Verification items for the finished model (mm, model axes). A direction names the side the tool comes from. Round coordinates to 2 decimals unless told otherwise and drop trailing zeros. Loops run counter-clockwise (first coordinate to the right, second up) from the corner with the lowest first, then second, coordinate; pieces in that order, holes last. Notation, with made-up numbers: (38, -3) - (42, -3) arc R21 cw to (42, 18) - close; hole circle Ø2 at (6.5, 73.5). An arc over 180 degrees is marked (long way). Use a Markdown table: item, result. Add a question column.
Autodesk Inventor part; units mm, degrees
ref_plane "YZ Plane" through (0, 0, 0) normal (1, 0, 0) x (0, 1, 0)
ref_plane "XZ Plane" through (0, 0, 0) normal (0, 1, 0) x (-1, 0, 0)
ref_plane "XY Plane" through (0, 0, 0) normal (0, 0, 1) x (1, 0, 0)
sketch "Sketch1" plane through (0, 0, 0) normal (0, 1, 0) x (-1, 0, 0)
  circle A0 centre (0, 0) radius 42.5
  arc A1 (55.6417, 25) -> (-55.6417, 25) centre (0, 0) ccw
  line L0 (0, 0) -> (0, -61)
  line L1 (0, 0) -> (0, 0)
  line L2 (0, 0) -> (0, -90.4875)
  line L3 (-117.5, 25) -> (-117.5, -25)
  line L4 (117.5, -25) -> (117.5, 25)
  line L5 (117.5, 25) -> (-117.5, -25) construction
  line L6 (-117.5, 25) -> (117.5, -25) construction
  line L7 (117.5, 25) -> (55.6417, 25)
  line L8 (-55.6417, 25) -> (-117.5, 25)
  line L9 (55.6417, -25) -> (117.5, -25)
  line L10 (-117.5, -25) -> (-55.6417, -25)
  arc A2 (-55.6417, -25) -> (55.6417, -25) centre (0, 0) ccw
  dimension "d0" = 85
  dimension "d29" = 61
  dimension "d46" = 235
  dimension "d47" = 50
extrude "Extrusion1" add sketch "Sketch1" along normal blind 5
sketch "Sketch2" plane through (0, 0, 0) normal (0, -1, 0) x (1, 0, 0)
  line L0 (-117.5, -25) -> (-117.5, 25)
  line L1 (-117.5, 0) -> (117.5, 0)
  line L2 (117.5, 25) -> (117.5, -25)
  arc A0 (55.6417, 25) -> (-55.6417, 25) centre (0, 0) ccw
  line L3 (0, 61) -> (0, -61)
  arc A1 (-55.6417, -25) -> (55.6417, -25) centre (0, 0) ccw
  circle A2 centre (-98.5, 11) radius 2
  line L4 (-117.5, 25) -> (-55.6417, 25)
  circle A3 centre (-78.5, 11) radius 2
  circle A4 centre (-98.5, -11) radius 2
  circle A5 centre (-78.5, -11) radius 2
  circle A6 centre (98.5, 11) radius 2
  circle A7 centre (78.5, 11) radius 2
  circle A8 centre (98.5, -11) radius 2
  circle A9 centre (78.5, -11) radius 2
  dimension "d51" = 4
  dimension "d52" = 19
  dimension "d53" = 14
  dimension "d54" = 4
  dimension "d55" = 20
hole "Hole1" at (-98.5, 0, 11) at (-78.5, 0, 11) at (-78.5, 0, -11) at (-98.5, 0, -11) at (78.5, 0, 11) at (98.5, 0, 11) at (98.5, 0, -11) at (78.5, 0, -11) direction (0, 1, 0) diameter 3.242 depth 11.8 tip angle 118
sketch "Sketch3" plane through (0, 0, 0) normal (0, -1, 0) x (1, 0, 0)
  circle A0 centre (0, 0) radius 51
  circle A1 centre (0, 51) radius 2
  circle A2 centre (-44.1673, 25.5) radius 2
  circle A3 centre (-44.1673, -25.5) radius 2
  circle A4 centre (0, -51) radius 2
  circle A5 centre (44.1673, -25.5) radius 2
  circle A6 centre (44.1673, 25.5) radius 2
  dimension "d33" = 102
  dimension "d34" = 4
  dimension "d37" = 360
hole "Hole2" at (0, 0, 51) at (44.1673, 0, 25.5) at (44.1673, 0, -25.5) at (0, 0, -51) at (-44.1673, 0, -25.5) at (-44.1673, 0, 25.5) direction (0, 1, 0) diameter 3.242 depth 11.8 tip angle 118
fillet "Fillet2" radius 5 8 edges at (-117.5, 2.5, -25) (-55.6417, 2.5, -25) (117.5, 2.5, -25) (55.6417, 2.5, -25) (117.5, 2.5, 25) (55.6417, 2.5, 25) (-55.6417, 2.5, 25) (-117.5, 2.5, 25)
properties part number "Head Thing (metal)"
Q1. Section check C-C on x = 4.5. Record the cut outline in (y, z), plus the area to 3 significant figures.
Q2. Section check D-D on x = -94.5. Record the cut outline in (y, z), plus the area to 3 significant figures.
Q3. Set-up check for faces 1 (the face through (-86, 2, 25)), 2 (the face through (85, 2, 25)), 3 (the face through (-85, 2, -25)): record each of +Z, -Z, +X, -X, +Y, -Y from which the full face is reachable in a straight line by a thin tool's end or side.
Q4. Section check B-B on y = 3.25. State how many separate pieces and enclosed holes the cut face has, plus the area to 3 significant figures.
Q5. Go/stop test with flat-tipped pins: pin 1 Ø1.9 at (x, z) = (-78.5, -11) entering from -Y; pin 2 Ø2.5 at (x, y) = (-76, 2.5) entering from -Z; pin 3 Ø1 at (x, y) = (-23, 3.5) entering from -Z; pin 4 Ø2.5 at (x, y) = (93, 1.5) entering from +Z. Record where each tip stops, or that it passes through.
Q6. Thickness scan on line 1 along Z through (x, y) = (98.5, 1.25); line 2 along Z through (x, y) = (0, 1.35); line 3 along X through (y, z) = (1.8, -11). Record the ranges inside material, lowest first.
Q7. Section check A-A on z = 0. Record the cut outline in (x, y), plus the area to 3 significant figures.
Determined:
| question | item | result |
|---|---|---|
| 1 | outline | (0, -60.83) - (5, -60.83) - (5, -42.26) - (0, -42.26) - close; (0, 42.26) - (5, 42.26) - (5, 60.83) - (0, 60.83) - close |
| 1 | area | 186 mm² |
| 2 | outline | (0, -25) - (5, -25) - (5, 25) - (0, 25) - close |
| 2 | area | 250 mm² |
| 3 | face 1 | +Z, -X, +Y, -Y |
| 3 | face 2 | +Z, +X, +Y, -Y |
| 3 | face 3 | -Z, -X, +Y, -Y |
| 4 | separate pieces | 1 |
| 4 | enclosed holes | 15 |
| 4 | area | 11,700 mm² |
| 5 | pin 1 | passes through |
| 5 | pin 2 | stops at z = -25 |
| 5 | pin 3 | stops at z = -56.7 |
| 5 | pin 4 | stops at z = 25 |
| 6 | line 1 | z = -25 to -12.62, -9.38 to 9.38, 12.62 to 25 |
| 6 | line 2 | z = -61 to -52.62, -49.38 to -42.5, 42.5 to 49.38, 52.62 to 61 |
| 6 | line 3 | x = -117.5 to -100.12, -96.88 to -80.12, -76.88 to -41.05, 41.05 to 76.88, 80.12 to 96.88, 100.12 to 117.5 |
| 7 | outline | (-117.5, 0) - (-42.5, 0) - (-42.5, 5) - (-117.5, 5) - close; (42.5, 0) - (117.5, 0) - (117.5, 5) - (42.5, 5) - close |
| 7 | area | 750 mm² |
